Answer from the drawing. Dimensions are ordinates in mm from the lowest x, y and z of the part. Give positions to 0.01 mm unless a question says otherwise; leave off trailing zeros. Order: outer loops, then holes, each group sorted by start corner. A loop starts at its lowest first (then second) coordinate and runs counter-clockwise, first axis right, second up. Notation, with made-up numbers: (84, -19) - (140, -19) arc R17 ccw to (140, 0) - close; hole circle Ø9 at (1.25, 65.25). An arc over 180 degrees is marked (long way). Write each question's results on one line, items separated by ' | '.
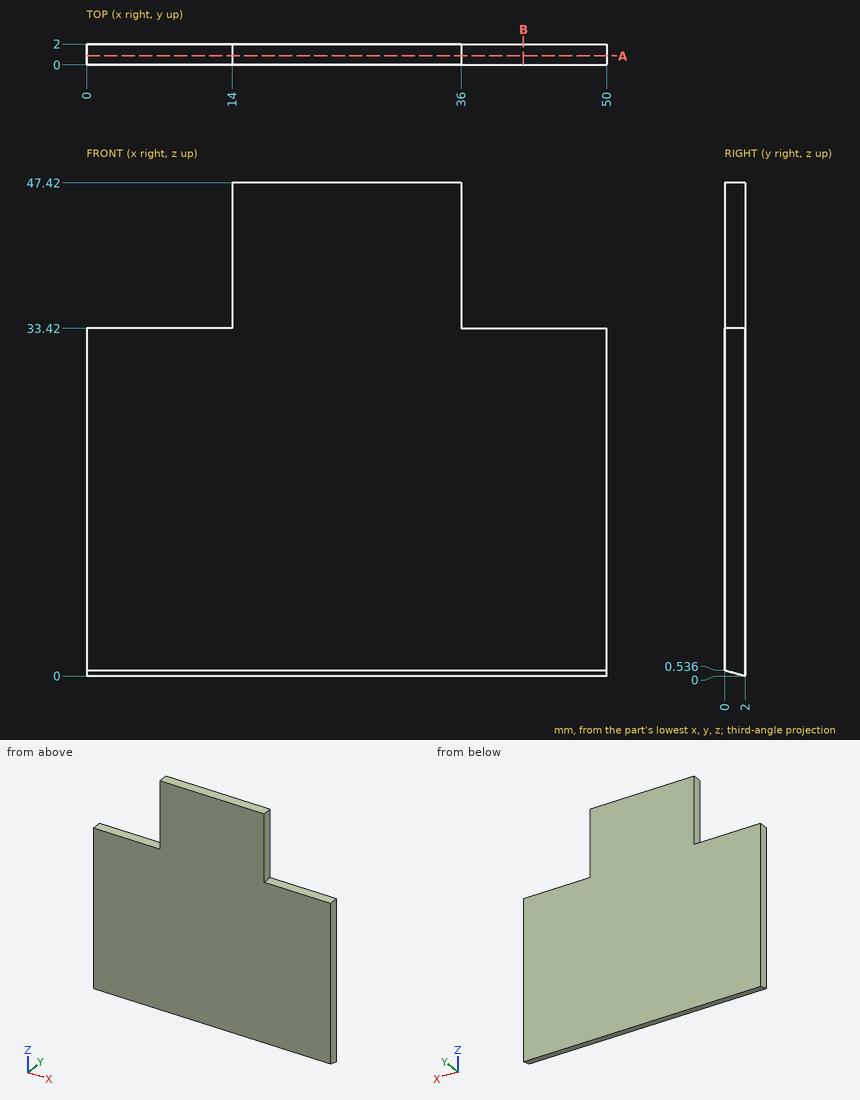
1. A cutting plane is placed at B-B, the plane x = 42. Write down the section's boundary in (y, z).
Answer list:
outline: (0, 0.54) - (2, 0) - (2, 33.42) - (0, 33.42) - close
2. A cutting plane is placed at A-A, the plane y = 0.85. Write down the section's boundary in (x, z).
Answer list:
outline: (0, 0.31) - (50, 0.31) - (50, 33.42) - (36, 33.42) - (36, 47.42) - (14, 47.42) - (14, 33.42) - (0, 33.42) - close
3. Straight lines are drawn through the part: line 1 (X direction, y = 0.5, z = 35); line 2 (Z direction, x = 13.5, y = 0.55); line 3 (Z direction, x = 42.5, y = 1.75). For each, find the intervals that lie inside material, in ascending order. Write a range as [from, to].
Answer list:
line 1: [14, 36] | line 2: [0.39, 33.42] | line 3: [0.07, 33.42]
4. Given P1, Ø1, axis at x = 9.5, y = 1, coming from the +Z side; P2, Ø0.6, axis at y = 0.5, z = 38, coming from the -X side, each flat-ended and moving along its own axis, determine where each tip first touches the part or whether it passes through.
Answer list:
P1: z = 33.42 | P2: x = 14
